Can you work these out from the model? Positions are in its coordinate system, mm. Give positions to 0.01 mm unless a question says otherwise; leave off trailing zeros. Loops run counter-clockwise (first coordinate to the right, second up) from the corner with the lowest first, then second, coordinate; pieces in that order, holes last. Notation, with made-up numbers: M 76.5,-15.75 L 91.5,-15.75 A22 ccw 91.5,12.25 Z; hole C 60.25,-23.5 d3. An arc over 180 degrees is marked long. Put each result on its own line as item: value. Start each with the question number.
1) Imagine slicing it at A-A (x = 50.8). Write out the boundary of the cut face in (y, z) (3 decimals), then the cut area to 3 significant figures.
2) If we mould it in two halves opening along X, with no side actions, what happens to faces 1 (the cylindrical face through (22.253, 1.256, 9.392)), 2 (the flat face through (-5, 4, 0)), 3 (the cylindrical face through (-146.05, 143.41, 9.39)), 4 (the flat face through (355.6, -4, 9))? For each: +X half, -X half, draft (parallel to the pull), parting line (faces both ways), or undercut.
3) For P1, Ø10.5, axis at x = 193.5, y = 208.28, coming from the -Z side, with a flat end and sliding along its axis, tell me the tip position at first contact or that it passes through.
4) Imagine slicing it at B-B (y = 0). Write out the boundary of the cut face in (x, z) (3 decimals), then the cut area to 3 significant figures.
5) Please list where these lines run through material, in increasing order: line 1 along Y through (x, z) = (258.5, 2.5); line 2 along Y through (x, z) = (-154, 1.25); line 3 along X through (y, z) = (2.5, 11.25). Write a range as from..to.
from build123d import *

# Parameters (mm, degrees)
F0_W     = 711.2
F0_H     = 609.6
F0_R     = 28.575
F1_DEPTH = 19.05
F3_D     = 17.85874


with BuildPart() as f1:
    # F0 (on Top) → F1 (new body)
    with BuildSketch(Plane.XY):
        Rectangle(F0_W, F0_H)
        with Locations((50.8, 0)):
            Circle(F0_R, mode=Mode.SUBTRACT)
    extrude(amount=F1_DEPTH)

    # F3 (through all)
    with Locations(Plane.XY.offset(19.05)):
        with Locations((-153.1352670464, 148.8440036774), (-91.9009929177, -208.2799971104), (257.6402368968, -144.7799950838), (193.5009929177, 208.2799971104)):
            Hole(F3_D / 2)


solid = f1.part
Recorded:
1. outline: M -304.8,0 L -28.575,0 L -28.575,19.05 L -304.8,19.05 Z; M 28.575,0 L 304.8,0 L 304.8,19.05 L 28.575,19.05 Z
1. area: 10,500 mm²
2. face 1: undercut
2. face 2: draft
2. face 3: undercut
2. face 4: +X half
3. P1: through
4. outline: M -355.6,0 L 22.225,0 L 22.225,19.05 L -355.6,19.05 Z; M 79.375,0 L 355.6,0 L 355.6,19.05 L 79.375,19.05 Z
4. area: 12,500 mm²
5. line 1: -304.8..-153.67, -135.89..304.8
5. line 2: -304.8..139.96, 157.73..304.8
5. line 3: -355.6..22.33, 79.27..355.6
